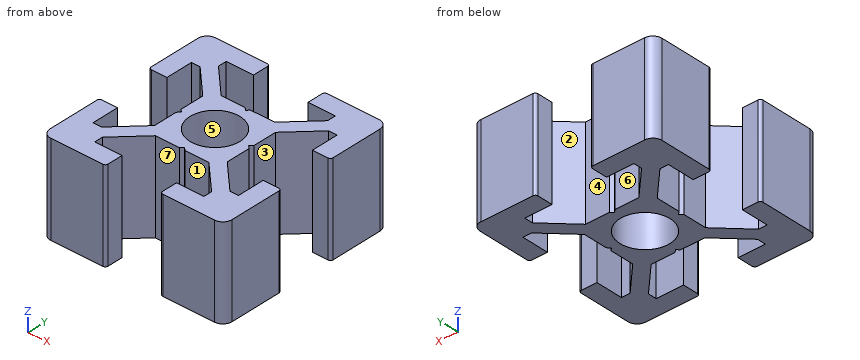
Autodesk Inventor part; units mm, degrees
ref_plane "Startebene" through (0, 0, 0) normal (0, 0, 1) x (1, 0, 0)
ref_plane "Endebene" through (0, 0, 320) normal (0, 0, 1) x (1, 0, 0)
ref_plane "Startebene1" through (0, 0, 0) normal (0, 0, 1) x (1, 0, 0)
ref_plane "Startebene" through (0, 0, 0) normal (0, 0, 1) x (1, 0, 0)
ref_plane "Endebene" through (0, 0, 320) normal (0, 0, 1) x (1, 0, 0)
ref_plane "Startebene1" through (0, 0, 0) normal (0, 0, 1) x (1, 0, 0)
ref_plane "Endebene1" through (0, 0, 10) normal (0, 0, 1) x (1, 0, 0)
ref_plane "Startebene2" through (0, 0, 0) normal (0, 0, 1) x (1, 0, 0)
ref_plane "Endebene2" through (0, 0, 10) normal (0, 0, 1) x (1, 0, 0)
sketch "Skizze" plane through (0, 0, 0) normal (0, 0, 1) x (1, 0, 0)
  line L0 (-10, 9) -> (-10, 3.3)
  arc A0 (-10, 3.3) -> (-9.7, 3) centre (-9.7, 3.3) ccw
  line L1 (-9.7, 3) -> (-8, 3)
  line L2 (-8, 3) -> (-8, 6)
  line L3 (-8, 6) -> (-7.0607, 6)
  line L4 (-7.0607, 6) -> (-4, 2.9393)
  line L5 (-4, 2.9393) -> (-4, 0.3)
  line L6 (-4, 0.3) -> (-3.7, 0)
  line L7 (-3.7, 0) -> (-4, -0.3)
  line L8 (-4, -0.3) -> (-4, -2.9393)
  line L9 (-4, -2.9393) -> (-7.0607, -6)
  line L10 (-7.0607, -6) -> (-8, -6)
  line L11 (-8, -6) -> (-8, -3)
  line L12 (-8, -3) -> (-9.7, -3)
  arc A1 (-9.7, -3) -> (-10, -3.3) centre (-9.7, -3.3) ccw
  line L13 (-10, -3.3) -> (-10, -9)
  arc A2 (-10, -9) -> (-9, -10) centre (-9, -9) ccw
  line L14 (-9, -10) -> (-3.3, -10)
  arc A3 (-3.3, -10) -> (-3, -9.7) centre (-3.3, -9.7) ccw
  line L15 (-3, -9.7) -> (-3, -8)
  line L16 (-3, -8) -> (-6, -8)
  line L17 (-6, -8) -> (-6, -7.0607)
  line L18 (-6, -7.0607) -> (-2.9393, -4)
  line L19 (-2.9393, -4) -> (-0.3, -4)
  line L20 (-0.3, -4) -> (0, -3.7)
  line L21 (0, -3.7) -> (0.3, -4)
  line L22 (0.3, -4) -> (2.9393, -4)
  line L23 (2.9393, -4) -> (6, -7.0607)
  line L24 (6, -7.0607) -> (6, -8)
  line L25 (6, -8) -> (3, -8)
  line L26 (3, -8) -> (3, -9.7)
  arc A4 (3, -9.7) -> (3.3, -10) centre (3.3, -9.7) ccw
  line L27 (3.3, -10) -> (9, -10)
  arc A5 (9, -10) -> (10, -9) centre (9, -9) ccw
  line L28 (10, -9) -> (10, -3.3)
  arc A6 (10, -3.3) -> (9.7, -3) centre (9.7, -3.3) ccw
  line L29 (9.7, -3) -> (8, -3)
  line L30 (8, -3) -> (8, -6)
  line L31 (8, -6) -> (7.0607, -6)
  line L32 (7.0607, -6) -> (4, -2.9393)
  line L33 (4, -2.9393) -> (4, -0.3)
  line L34 (4, -0.3) -> (3.7, 0)
  line L35 (3.7, 0) -> (4, 0.3)
  line L36 (4, 0.3) -> (4, 2.9393)
  line L37 (4, 2.9393) -> (7.0607, 6)
  line L38 (7.0607, 6) -> (8, 6)
  line L39 (8, 6) -> (8, 3)
  line L40 (8, 3) -> (9.7, 3)
  arc A7 (9.7, 3) -> (10, 3.3) centre (9.7, 3.3) ccw
  line L41 (10, 3.3) -> (10, 9)
  arc A8 (10, 9) -> (9, 10) centre (9, 9) ccw
  line L42 (9, 10) -> (3.3, 10)
  arc A9 (3.3, 10) -> (3, 9.7) centre (3.3, 9.7) ccw
  line L43 (3, 9.7) -> (3, 8)
  line L44 (3, 8) -> (6, 8)
  line L45 (6, 8) -> (6, 7.0607)
  line L46 (6, 7.0607) -> (2.9393, 4)
  line L47 (2.9393, 4) -> (0.3, 4)
  line L48 (0.3, 4) -> (0, 3.7)
  line L49 (0, 3.7) -> (-0.3, 4)
  line L50 (-0.3, 4) -> (-2.9393, 4)
  line L51 (-2.9393, 4) -> (-6, 7.0607)
  line L52 (-6, 7.0607) -> (-6, 8)
  line L53 (-6, 8) -> (-3, 8)
  line L54 (-3, 8) -> (-3, 9.7)
  arc A10 (-3, 9.7) -> (-3.3, 10) centre (-3.3, 9.7) ccw
  line L55 (-3.3, 10) -> (-9, 10)
  arc A11 (-9, 10) -> (-10, 9) centre (-9, 9) ccw
  circle A12 centre (0, 0) radius 2.75
  dimension "d2" = 5.5
  dimension "d3" = 10
  dimension "d4" = 10
  dimension "d5" = 5.7
  dimension "d6" = 5.7
  dimension "d7" = 1.7
  dimension "d8" = 3
  dimension "d9" = 0.3
  dimension "d10" = 90
  dimension "d11" = 45
  dimension "d12" = 45
  dimension "d13" = 45
  dimension "d14" = 90
  dimension "d15" = 90
  dimension "d16" = 45
  dimension "d17" = 45
  dimension "d18" = 45
  dimension "d19" = 45
  dimension "d20" = 90
  dimension "d21" = 90
  dimension "d22" = 45
  dimension "d23" = 45
  dimension "d24" = 90
  dimension "d25" = 90
  dimension "d26" = 90
  dimension "d27" = 90
  dimension "d28" = 90
  dimension "d29" = 90
  dimension "d30" = 90
  dimension "d31" = 90
  dimension "d32" = 90
  dimension "d33" = 90
  dimension "d34" = 90
  dimension "d35" = 90
  dimension "d36" = 90
  dimension "d37" = 90
  dimension "d38" = 90
  dimension "d39" = 4
  dimension "d40" = 6
  dimension "d41" = 13
  dimension "d42" = 14
  dimension "d43" = 16
  dimension "d44" = 18
  dimension "d45" = 3
  dimension "d46" = 9
  dimension "d47" = 7
  dimension "d48" = 1
  dimension "d49" = 7
  dimension "d50" = 1.5
  dimension "d51" = 1.8663
  dimension "d52" = 3.3663
  dimension "d53" = 1.5
  dimension "d54" = 1.8663
  dimension "d55" = 3.3663
  dimension "d56" = 4
  dimension "d57" = 10.8187
  dimension "d58" = 1.9092
  dimension "d59" = 5
  dimension "d60" = 13
  dimension "d61" = 13
  dimension "d62" = 16.0513
  dimension "d63" = 3.3234
  dimension "d64" = 14
  dimension "d65" = 12.685
extrude "Körper" add sketch "Skizze" along normal up to surface (10 mm away) from surface at 0
sketch "Skizze13" plane through (0, 0, 0) normal (0, 0, 1) x (1, 0, 0)
  line L0 (0, 0) -> (10, 0)
ref_plane "Arbeitsebene12" through (0, 0, 0) normal (0, -1, 0) x (1, 0, 0)
sketch "Skizze14" plane through (0, 0, 0) normal (0, -1, 0) x (1, 0, 0)
  line L0 (-2, 0) -> (12, 0)
  line L1 (-2, 10) -> (12, 10)
  dimension "d80" = 10
equation "\"G_OFFSET_START\" = 0"
equation "\"G_OFFSET_END\" = 0"
equation "\"G_L\" = d80"
equation "\"G_OFFSET_START1\" = 0"
equation "\"G_OFFSET_END1\" = 0"
equation "\"G_OFFSET_START2\" = 0"
equation "\"G_OFFSET_END2\" = 0"
properties part number "Alu Profil 20x20 - AP2020" material "Aluminium 6061"
Here's how the part is built. I have some questions about the finished solid (model axes, mm). Face numbers are marked on the shaded views. A direction names the side the tool comes from. Coordinates: 2 decimals unless noted, no trailing zeros. Write each loop counter-clockwise with the first axis right and the second up, starting at its lowest first coordinate (ties: lowest second). Pieces come first, ordered by that corner, then holes.
1) Thinking about a two-plate mould opening in Y: for the marked faces 5, 6 and 7, which applies, +Y half, -Y half, draft (parallel to the pull), parting line (faces both ways), or undercut?
Filled in:
face 5: undercut
face 6: +Y half
face 7: -Y half
2) Which directions (+Z, -Z, +X, -X, +Y, -Y) give clear straight access to the entire face, cutting with the end or side of a thin tool? Please do the marked faces 1, 2, 3 and 4.
Filled in:
face 1: +Z, -Z, -Y
face 2: +Z, -Z
face 3: +Z, -Z, +X
face 4: +Z, -Z, +Y
3) If we section it at A-A (x = -5.5): List the corners of the cut face in (y, z) for me, plus the area to 3 significant figures.
Filled in:
outline: (-10, 0) - (-8, 0) - (-8, 10) - (-10, 10) - close; (-6.56, 0) - (-4.44, 0) - (-4.44, 10) - (-6.56, 10) - close; (4.44, 0) - (6.56, 0) - (6.56, 10) - (4.44, 10) - close; (8, 0) - (10, 0) - (10, 10) - (8, 10) - close
area: 82.4 mm2
4) If we section it at B-B (y = 2): List the corners of the cut face in (x, z) for me.
Filled in:
outline: (-4, 0) - (-1.89, 0) - (-1.89, 10) - (-4, 10) - close; (1.89, 0) - (4, 0) - (4, 10) - (1.89, 10) - close
5) If we section it at C-C (x = 6.5): List the corners of the cut face in (y, z) for me, plus the area to 3 significant figures.
Filled in:
outline: (-10, 0) - (-5.44, 0) - (-5.44, 10) - (-10, 10) - close; (5.44, 0) - (10, 0) - (10, 10) - (5.44, 10) - close
area: 91.2 mm2
6) If I drill on line 1 (X direction, y = -8.75, z = 8.25); line 2 (X direction, y = 3.25, z = 9), over which ranges is the centre line in solid material (lowest first)?
Filled in:
line 1: x = -10 to -3, 3 to 10
line 2: x = -10 to -8, -4.31 to 4.31, 8 to 10
